from build123d import *

# Parameters (mm, degrees)
SKETCH_1_W          = 20
SKETCH_1_H          = 10.5
EXTRUDE_1_DEPTH     = 6.5
SKETCH_2_R          = 1.25
CUT_EXTRUDE_1_DEPTH = 6.5
SKETCH_3_W          = 4.44626532
SKETCH_3_H          = 1.008872475
SKETCH_3_W_2        = 5
SKETCH_3_W_3        = 3.65317203
CUT_EXTRUDE_2_DEPTH = 6.5
CHAMFER_1_SIZE      = 0.45
SKETCH_4_W          = 10.31021277
SKETCH_4_H          = 1.008783122
CUT_EXTRUDE_3_DEPTH = 6.5
CHAMFER_2_SIZE      = 0.75
SKETCH_5_W          = 2
SKETCH_5_H          = 1.4
EXTRUDE_2_DEPTH     = 4
FILLET_1_R          = 0.5


with BuildPart() as part:
    # 스케치1 → 보스-돌출1 (new body)
    with BuildSketch(Plane(origin=(0, 0, 0), x_dir=(1, 0, 0), z_dir=(0, 1, 0))):
        Rectangle(SKETCH_1_W, SKETCH_1_H)
    extrude(amount=EXTRUDE_1_DEPTH)

    # 스케치2 → 컷-돌출1 (cut)
    with BuildSketch(Plane(origin=(0, 6.5, 0), x_dir=(1, 0, 0), z_dir=(0, 1, 0))):
        with Locations(Location((-4.75, -2.1, 0), (0, 0, 270))):
            Circle(SKETCH_2_R)
        with Locations(Location((4.75, -2.1, 0), (0, 0, 270))):
            Circle(SKETCH_2_R)
    extrude(amount=-CUT_EXTRUDE_1_DEPTH, mode=Mode.SUBTRACT)

    # 스케치3 → 컷-돌출2 (cut)
    with BuildSketch(Plane(origin=(0, 6.5, 0), x_dir=(1, 0, 0), z_dir=(0, 1, 0))):
        with Locations((-9.22313266, -5.304436238)):
            Rectangle(SKETCH_3_W, SKETCH_3_H)
        with Locations((0, -5.304436238)):
            Rectangle(SKETCH_3_W_2, SKETCH_3_H)
        with Locations((8.826586015, -5.304436238)):
            Rectangle(SKETCH_3_W_3, SKETCH_3_H)
    extrude(amount=-CUT_EXTRUDE_2_DEPTH, mode=Mode.SUBTRACT)

    # 모따기1
    chamfer_1_edges = [part.edges().sort_by_distance(p)[0] for p in [
        (7, 3.25, 5.25),
        (2.5, 3.25, 5.25),
        (-2.5, 3.25, 5.25),
        (-7, 3.25, 5.25),
    ]]
    chamfer(chamfer_1_edges, length=CHAMFER_1_SIZE - 0.0001)  # a hair under: the kernel refuses the full size

    # 스케치4 → 컷-돌출3 (cut)
    with BuildSketch(Plane(origin=(0, 6.5, 0), x_dir=(1, 0, 0), z_dir=(0, 1, 0))):
        with Locations((5.155106385, 5.004391561)):
            Rectangle(SKETCH_4_W, SKETCH_4_H)
    extrude(amount=-CUT_EXTRUDE_3_DEPTH, mode=Mode.SUBTRACT)

    # 모따기2
    chamfer_2_edges = [part.edges().sort_by_distance(p)[0] for p in [
        (0, 3.25, -5.25),
    ]]
    chamfer(chamfer_2_edges, length=CHAMFER_2_SIZE - 0.0001)  # a hair under: the kernel refuses the full size

    # 스케치5 → 보스-돌출2 (add)
    with BuildSketch(Plane(origin=(0, 5.25, 0), x_dir=(1, 0, 0), z_dir=(0, 1, 0))):
        with Locations((-3, 5.95)):
            Rectangle(SKETCH_5_W, SKETCH_5_H)
    extrude(amount=-EXTRUDE_2_DEPTH)

    # 필렛1
    fillet_1_edges = [part.edges().sort_by_distance(p)[0] for p in [
        (-4, 3.25, -6.65),
        (-2, 3.25, -6.65),
    ]]
    fillet(fillet_1_edges, radius=FILLET_1_R)


solid = part.part
Here's how the part is built. I have some questions about the finished solid (model axes, mm). A direction names the side the tool comes from. Give positions to 0.01 mm unless a question says otherwise; leave off trailing zeros. Order: outer loops, then holes, each group sorted by start corner. A loop starts at its lowest first (then second) coordinate and runs counter-clockwise, first axis right, second up. Notation, with made-up numbers: M 25,81.25 L 62,81.25 A29 ccw 62,106.25 Z; hole C -40,12 d2. An arc over 180 degrees is marked long. Answer as a JSON object with one key per item and string values. Group by question number.
1) We'd pull the mould along X, two halves only. Please class faces 4 (the cylindrical face through (-5.97, 3.3, 1.83)), 5 (the cylindrical face through (3.53, 3.3, 1.83)), 6 (the flat face through (-10, 3, 0)), 7 (the flat face through (-9, 3, 4.8)): pulls with the +X half, pulls with the -X half, needs draft (parallel to the pull), parting line crosses it, or undercut.
2) Suppose I cut it at A-A, the plane x = 4.75. Write out the boundary of the cut face in (y, z).
3) Suppose I cut it at C-C, the plane z = 2.1. Write out the boundary of the cut face in (x, y).
4) Please list where these lines run through material, in increasing order: L1, parallel to X at y = 4.5, z = 2.1; L2, parallel to X at y = 0.5, z = 1.5; L3, parallel to Z at x = 1.5, y = 1. Write a range as [from, to].
5) Suppose I cut it at B-B, the plane y = 2. Count the separate pieces of the cut face and the enclosed holes in it, plus the area to 3 significant figures.
6) On a 3-axis mill with a long thin cutter (end or side, diameter ignored), from which of +Z, -Z, +X, -X, +Y, -Y can I reach the whole of each face in a straight line? I mean faces 1 (the flat face through (0, 3, 4.8)), 2 (the flat face through (-2, 3, -6)), 3 (the flat face through (-3, 1.25, -6)). Say none if no direction works.
7) Suppose I cut it at D-D, the plane x = -4.75. Write out the boundary of the cut face in (y, z), plus the area to 3 significant figures.
8) I'm going to push flat-ended pins straight in: pin 1 Ø1 at (y, z) = (3.5, -6) entering from +X; pin 2 Ø3 at (x, z) = (-4.75, 2.1) entering from -Y; pin 3 Ø2.5 at (x, y) = (-8, 2.5) entering from +Z; pin 4 Ø2 at (x, y) = (3.5, 4.5) entering from -Z. Where does each tip first touch, or does it pass through?
Results found:
{
 "1": {"face 4": "undercut", "face 5": "undercut", "face 6": "pulls with the -X half", "face 7": "needs draft"},
 "2": {"outline": "M 0,-4.5 L 6.5,-4.5 L 6.5,0.85 L 0,0.85 Z; M 0,3.35 L 6.5,3.35 L 6.5,5.25 L 0,5.25 Z"},
 "3": {"outline": "M -10,0 L -6,0 L -6,6.5 L -10,6.5 Z; M -3.5,0 L 3.5,0 L 3.5,6.5 L -3.5,6.5 Z; M 6,0 L 10,0 L 10,6.5 L 6,6.5 Z"},
 "4": {"L1": "[-10, -6], [-3.5, 3.5], [6, 10]", "L2": "[-10, -5.85], [-3.65, 3.65], [5.85, 10]", "L3": "[-4.5, 4.8]"},
 "5": {"separate pieces": "1", "enclosed holes": "2", "area": "190 mm²"},
 "6": {"face 1": "+Z, +Y, -Y", "face 2": "-Z, +X, +Y, -Y", "face 3": "-Z, +X, -X, -Y"},
 "7": {"outline": "M 0,-5.25 L 6.5,-5.25 L 6.5,0.85 L 0,0.85 Z; M 0,3.35 L 6.5,3.35 L 6.5,5.25 L 0,5.25 Z", "area": "52.0 mm²"},
 "8": {"pin 1": "x = -2", "pin 2": "y = 0", "pin 3": "z = 5.05", "pin 4": "z = -4.5"}
}
